from build123d import *

# Parameters (mm, degrees)
F0_W     = 177.8
F0_H     = 50.8
F1_DEPTH = 25.4
F2_R     = 12.7
F3_DEPTH = 25.4
F5_DEPTH = 6.35
F6_R     = 6.35
F7_R     = 12.7
F8_R     = 6.35


with BuildPart() as f1:
    # F0 (on Top) → F1 (new body)
    with BuildSketch(Plane.XY):
        with Locations((-88.9, 101.6)):
            Rectangle(F0_W, F0_H)
        Polygon((0, 76.2), (0, 0), (228.6, 0), (228.6, 203.2), (0, 203.2), (0, 127), align=None)
    extrude(amount=F1_DEPTH)

    # F2 (on face) → F3 (cut)
    with BuildSketch(Plane.XY.offset(25.4)):
        with Locations((-152.4, 101.6)):
            Circle(F2_R)
    extrude(amount=-F3_DEPTH, mode=Mode.SUBTRACT)

    # F4 (on face) → F5 (cut)
    with BuildSketch(Plane.XY.offset(25.4)):
        Polygon((12.699994, 76.2), (12.699994, 12.699994), (215.900006, 12.699994), (215.900006, 190.500006), (12.699994, 190.500006), (12.699994, 127), align=None)
        Polygon((25.399994, 76.2), (25.399994, 127), (25.399994, 177.800006), (203.200006, 177.800006), (203.200006, 25.399994), (25.399994, 25.399994), align=None, mode=Mode.SUBTRACT)
    extrude(amount=-F5_DEPTH, mode=Mode.SUBTRACT)

    # F6
    f6_edges = [f1.edges().sort_by_distance(p)[0] for p in [
        (12.699994, 190.500006, 22.225),
        (215.900006, 190.500006, 22.225),
        (12.699994, 12.699994, 22.225),
        (215.900006, 12.699994, 22.225),
    ]]
    fillet(f6_edges, radius=F6_R)

    # F7
    f7_edges = [f1.edges().sort_by_distance(p)[0] for p in [
        (0, 203.2, 12.7),
        (0, 127, 12.7),
        (-177.8, 127, 12.7),
        (-177.8, 76.2, 12.7),
        (228.6, 203.2, 12.7),
        (228.6, 0, 12.7),
        (0, 0, 12.7),
    ]]
    fillet(f7_edges, radius=F7_R)

    # F8
    f8_edges = [f1.edges().sort_by_distance(p)[0] for p in [
        (0, 76.2, 12.7),
    ]]
    fillet(f8_edges, radius=F8_R)


solid = f1.part
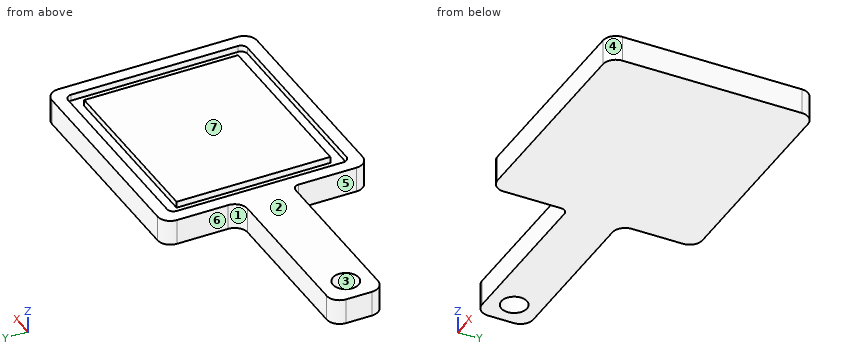
Can you work these out from the model? Positions are in its coordinate system, mm. Face numbers are marked on the shaded views. A direction names the side the tool comes from. Give positions to 0.01 mm unless a question says otherwise; leave off trailing zeros. Order: outer loops, then holes, each group sorted by start corner. A loop starts at its lowest first (then second) coordinate and runs counter-clockwise, first axis right, second up. Notation, with made-up numbers: (30, 5.5) - (34, 5.5) arc R11 cw to (34, 16.5) - close; hole circle Ø3 at (51, 48). An arc over 180 degrees is marked (long way). Write each question's results on one line, items separated by ' | '.
1) Please list where these lines run through material, in increasing order: line 1 along X through (y, z) = (38, 24); line 2 along Y through (x, z) = (-152.4, 14.5); line 3 along X through (y, z) = (67.5, 7.25). Write a range as [from, to].
Final values:
line 1: x = [0, 12.7], [25.4, 203.2], [215.9, 228.6] | line 2: y = [76.2, 88.9], [114.3, 127] | line 3: x = [0, 228.6]
2) Suppose I cut it at D-D, the plane x = 197. Write out the boundary of the cut face in (y, z), then the cut area to 3 significant figures.
Final values:
outline: (0, 0) - (203.2, 0) - (203.2, 25.4) - (190.5, 25.4) - (190.5, 19.05) - (177.8, 19.05) - (177.8, 25.4) - (25.4, 25.4) - (25.4, 19.05) - (12.7, 19.05) - (12.7, 25.4) - (0, 25.4) - close | area: 5,000 mm^2
3) On a 3-axis mill with a long thin cutter (end or side, diameter ignored), from which of +Z, -Z, +X, -X, +Y, -Y can I reach the whole of each face in a straight line? I mean the marked faces 5, 6 and 7. Say none if no direction works.
Final values:
face 5: +Z, -Z, -X, -Y | face 6: +Z, -Z, -X, +Y | face 7: +Z, +X, -X, +Y, -Y
4) If we mould it in two halves opening along Y, with no side actions, what happens to the marked faces 1, 2, 3 and 4? For each: pulls with the +Y half, pulls with the -Y half, needs draft (parallel to the pull), parting line crosses it, or undercut.
Final values:
face 1: pulls with the +Y half | face 2: needs draft | face 3: undercut | face 4: pulls with the -Y half
5) Suppose I cut it at B-B, the plane x = -152.4. Write out the boundary of the cut face in (y, z).
Final values:
outline: (76.2, 0) - (88.9, 0) - (88.9, 25.4) - (76.2, 25.4) - close; (114.3, 0) - (127, 0) - (127, 25.4) - (114.3, 25.4) - close
6) I'm going to push flat-ended pins straight in: pin 1 Ø5 at (y, z) = (66, 22) entering from -X; pin 2 Ø3 at (x, y) = (47.5, 64.5) entering from -Z; pin 3 Ø12.5 at (x, z) = (-86.5, 18.5) entering from +Y; pin 4 Ø7 at (y, z) = (136.5, 23) entering from -X. Where does each tip first touch, or does it pass through?
Final values:
pin 1: stops at x = 0 | pin 2: stops at z = 0 | pin 3: stops at y = 127 | pin 4: stops at x = -1.91
7) Suppose I cut it at A-A, the plane y = 101.6. Write out the boundary of the cut face in (x, z).
Final values:
outline: (-177.8, 0) - (-165.1, 0) - (-165.1, 25.4) - (-177.8, 25.4) - close; (-139.7, 0) - (228.6, 0) - (228.6, 25.4) - (215.9, 25.4) - (215.9, 19.05) - (203.2, 19.05) - (203.2, 25.4) - (25.4, 25.4) - (25.4, 19.05) - (12.7, 19.05) - (12.7, 25.4) - (-139.7, 25.4) - close
8) Suppose I cut it at C-C, the plane z = 8.5. Write out the boundary of the cut face in (x, y).
Final values:
outline: (-177.8, 88.9) arc R12.7 ccw to (-165.1, 76.2) - (-6.35, 76.2) arc R6.35 cw to (0, 69.85) - (0, 12.7) arc R12.7 ccw to (12.7, 0) - (215.9, 0) arc R12.7 ccw to (228.6, 12.7) - (228.6, 190.5) arc R12.7 ccw to (215.9, 203.2) - (12.7, 203.2) arc R12.7 ccw to (0, 190.5) - (0, 139.7) arc R12.7 cw to (-12.7, 127) - (-165.1, 127) arc R12.7 ccw to (-177.8, 114.3) - close; hole circle Ø25.4 at (-152.4, 101.6)
